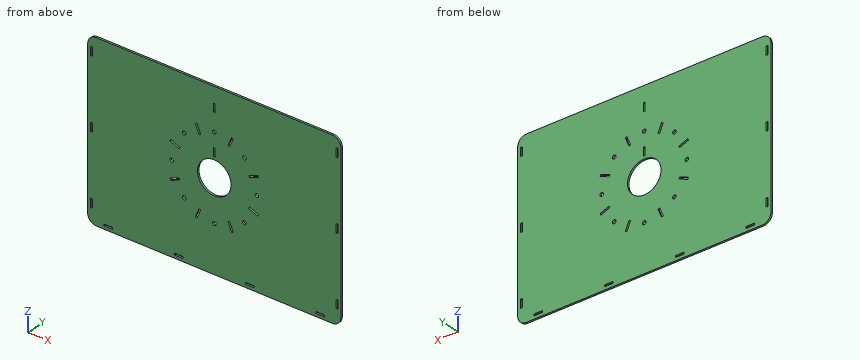
```python
from build123d import *

# Parameters (mm, degrees)
BOSS_EXTRUDE1_DEPTH = 3
CUT_EXTRUDE1_DEPTH  = 3
SKETCH3_R           = 27.5
CUT_EXTRUDE2_DEPTH  = 3
CIRPATTERN1_COUNT   = 8
SKETCH5_R           = 3
CUT_EXTRUDE4_DEPTH  = 3
CIRPATTERN2_COUNT   = 8
SKETCH6_W           = 14
SKETCH6_H           = 3
CUT_EXTRUDE7_DEPTH  = 3
SKETCH8_W           = 3
SKETCH8_H           = 14
CUT_EXTRUDE8_DEPTH  = 3
SKETCH10_W          = 3
SKETCH10_H          = 14
CUT_EXTRUDE9_DEPTH  = 3


with BuildPart() as part:
    # Sketch1 → Boss-Extrude1 (new body)
    with BuildSketch(Plane(origin=(0, 0, 0), x_dir=(1, 0, 0), z_dir=(0, 1, 0))):
        with BuildLine():
            Line((-193.857864376, -140), (193.857864376, -140))
            ThreePointArc((193.857864376, -140), (203.857864376, -135.857864376), (208, -125.857864376))
            Line((208, -125.857864376), (208, 133.857864376))
            ThreePointArc((208, 133.857864376), (203.857864376, 143.857864376), (193.857864376, 148))
            Line((193.857864376, 148), (-193.857864376, 148))
            ThreePointArc((-193.857864376, 148), (-203.857864376, 143.857864376), (-208, 133.857864376))
            Line((-208, 133.857864376), (-208, -125.857864376))
            ThreePointArc((-208, -125.857864376), (-203.857864376, -135.857864376), (-193.857864376, -140))
        make_face()
    extrude(amount=BOSS_EXTRUDE1_DEPTH)

    # Sketch2 → Cut-Extrude1 (cut)
    with BuildSketch(Plane(origin=(0, 3, 0), x_dir=(1, 0, 0), z_dir=(0, 1, 0))):
        Polygon((-31.227780816, 71.471989723), (-28.456142219, 72.62004002), (-22.333207301, 57.8379675), (-25.104845898, 56.689917202), align=None)
    cut_extrude1 = extrude(amount=-CUT_EXTRUDE1_DEPTH, mode=Mode.SUBTRACT)

    # Sketch3 → Cut-Extrude2 (cut)
    with BuildSketch(Plane(origin=(0, 3, 0), x_dir=(1, 0, 0), z_dir=(0, 1, 0))):
        Circle(SKETCH3_R)
    extrude(amount=-CUT_EXTRUDE2_DEPTH, mode=Mode.SUBTRACT)

    # CirPattern1: Cut-Extrude1 ×8 about axis
    cirpattern1_axis = Axis((0, 0, 0), (0, 1, 0))
    for i in range(1, CIRPATTERN1_COUNT):
        add(cut_extrude1.rotate(cirpattern1_axis, i * 360 / CIRPATTERN1_COUNT), mode=Mode.SUBTRACT)

    # Sketch5 → Cut-Extrude4 (cut)
    with BuildSketch(Plane(origin=(0, 3, 0), x_dir=(1, 0, 0), z_dir=(0, 1, 0))):
        with Locations((0, 70)):
            Circle(SKETCH5_R)
    cut_extrude4 = extrude(amount=-CUT_EXTRUDE4_DEPTH, mode=Mode.SUBTRACT)

    # CirPattern2: Cut-Extrude4 ×8 about axis
    cirpattern2_axis = Axis((0, 0, 0), (0, 1, 0))
    for i in range(1, CIRPATTERN2_COUNT):
        add(cut_extrude4.rotate(cirpattern2_axis, i * 360 / CIRPATTERN2_COUNT), mode=Mode.SUBTRACT)

    # Sketch6 → Cut-Extrude7 (cut)
    with BuildSketch(Plane(origin=(0, 3, 0), x_dir=(1, 0, 0), z_dir=(0, 1, 0))):
        with Locations((174, 141.5)):
            Rectangle(SKETCH6_W, SKETCH6_H)
        with Locations((-174, 141.5)):
            Rectangle(SKETCH6_W, SKETCH6_H)
        with Locations((58, 141.5)):
            Rectangle(SKETCH6_W, SKETCH6_H)
        with Locations((-58, 141.5)):
            Rectangle(SKETCH6_W, SKETCH6_H)
    extrude(amount=-CUT_EXTRUDE7_DEPTH, mode=Mode.SUBTRACT)

    # Sketch8 → Cut-Extrude8 (cut)
    with BuildSketch(Plane(origin=(0, 3, 0), x_dir=(1, 0, 0), z_dir=(0, 1, 0))):
        with Locations((201.5, 116)):
            Rectangle(SKETCH8_W, SKETCH8_H)
        with Locations((-201.5, 116)):
            Rectangle(SKETCH8_W, SKETCH8_H)
        with Locations((201.5, 0)):
            Rectangle(SKETCH8_W, SKETCH8_H)
        with Locations((-201.5, 0)):
            Rectangle(SKETCH8_W, SKETCH8_H)
        with Locations((201.5, -116)):
            Rectangle(SKETCH8_W, SKETCH8_H)
        with Locations((-201.5, -116)):
            Rectangle(SKETCH8_W, SKETCH8_H)
    extrude(amount=-CUT_EXTRUDE8_DEPTH, mode=Mode.SUBTRACT)

    # Sketch10 → Cut-Extrude9 (cut)
    with BuildSketch(Plane(origin=(0, 3, 0), x_dir=(1, 0, 0), z_dir=(0, 1, 0))):
        with Locations((0, -39)):
            Rectangle(SKETCH10_W, SKETCH10_H)
        with Locations((0, -107)):
            Rectangle(SKETCH10_W, SKETCH10_H)
    extrude(amount=-CUT_EXTRUDE9_DEPTH, mode=Mode.SUBTRACT)


solid = part.part
```
Check sheet for the modelled part. Datum: model origin and axes. Units: mm. Give positions to 0.01 mm unless a question says otherwise; leave off trailing zeros.
Item 1: Gauge pin test, flat ends, axial feed: pin 1 (1.5 mm diameter, centred on x = 202, y = 2, fed in from +Z); pin 2 (0.9 mm diameter, centred on x = -202, y = 1, fed in from +Z); pin 3 (0.9 mm diameter, centred on y = 2, z = -141.5, fed in from +X). Record the tip position at first contact, or that the pin passes through.
Item 2: Scan lines: L1, parallel to X at y = 0.65, z = 121; L2, parallel to X at y = 0.85, z = 0; L3, parallel to Z at x = -48, y = 0.3. Record each from-to range of solid material in increasing order.
Item 3: Cross-section at A-A (y = 0.65). Count the separate pieces of the cut face and the enclosed holes in it, and give its area (3 significant figures).
Report:
1. pin 1: stops at z = 137.91
1. pin 2: stops at z = 137.73
1. pin 3: stops at x = 206.03
2. L1: x = -208 to -203, -200 to 200, 203 to 208
2. L2: x = -208 to -203, -200 to -73, -67 to -27.5, 27.5 to 67, 73 to 200, 203 to 208
2. L3: z = -148 to -52.1, -46.9 to 46.9, 52.1 to 140
3. separate pieces: 1
3. enclosed holes: 29
3. area: 116,000 mm2
